For this review, use the dimensioned drawing (mm, ordinates from the lowest corner) and the shaded views. A direction names the side the tool comes from. Round coordinates to 2 decimals unless told otherwise and drop trailing zeros. Write each loop counter-clockwise with the first axis right and the second up, starting at its lowest first coordinate (ties: lowest second). Pieces come first, ordered by that corner, then holes. Notation, with made-up numbers: M 5,-21 L 57,-21 A17 cw 57,5 Z; hole C 70,34 d4. An arc over 180 degrees is marked long. Write each question's results on one line, items separated by ' | '. Start each with the question number.
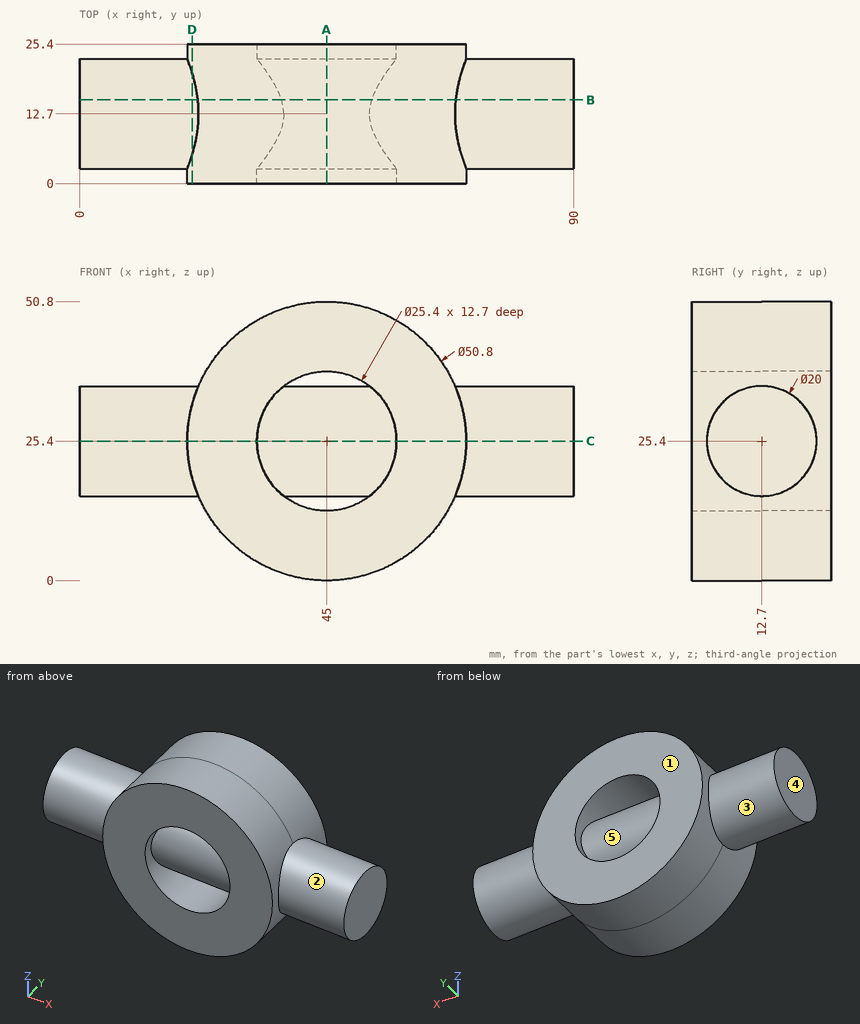
Item 1: We need section A-A on x = 45. State the section outline as (y, z) points, then the cut area to 3 significant figures.
Item 2: We need section C-C on z = 25.4. State the section outline as (x, y) points.
Item 3: For probe 1 along Z at (x, y) = (45, 22.75); probe 2 along Z at (x, y) = (45, 4); probe 3 along Z at (x, y) = (23, 17.75), list the stretches that pass through material, from the lowest coordinate up.
Item 4: We need section B-B on y = 15.25. State the section outline as (x, z) points, then the cut area to 3 significant figures.
Item 5: For the marked faces 1 and 2, list the 3-axis set-ups (+Z, -Z, +X, -X, +Y, -Y) from which the entire face can be reached by the end or side of a thin tool; tool diameter is ignored.
Item 6: Mouldability with a two-part tool opening along Z and no side actions: class the marked faces 3, 4 and 5 as pulls with the +Z half, pulls with the -Z half, needs draft (parallel to the pull), parting line crosses it, or undercut.
Item 7: We need section D-D on x = 20.5. State the section outline as (y, z) points, then the cut area to 3 significant figures.
Item 8: Insertion check: P1, Ø6, axis at y = 9.5, z = 8.5, coming from the +X side; P2, Ø23, axis at x = 45, z = 25.4, coming from the -Y side; P3, Ø6, axis at y = 10, z = 11, coming from the -X side. Each pin has a flat end and moves straight along its axis. Give the tip position at first contact, or say it passes through.
Numbers:
1) outline: M 0,0 L 25.4,0 L 25.4,12.7 L 0,12.7 Z; M 0,38.1 L 25.4,38.1 L 25.4,50.8 L 0,50.8 Z; C 12.7,25.4 d20 | area: 959 mm^2
2) outline: M 0,2.7 L 19.6,2.7 L 19.6,0 L 32.3,0 L 32.3,2.7 L 57.7,2.7 L 57.7,0 L 70.4,0 L 70.4,2.7 L 90,2.7 L 90,22.7 L 70.4,22.7 L 70.4,25.4 L 57.7,25.4 L 57.7,22.7 L 32.3,22.7 L 32.3,25.4 L 19.6,25.4 L 19.6,22.7 L 0,22.7 Z
3) probe 1: z = 0 to 12.7, 38.1 to 50.8 | probe 2: z = 0 to 12.7, 20.47 to 30.33, 38.1 to 50.8 | probe 3: z = 12.71 to 38.09
4) outline: M 0,15.73 L 21.51,15.73 A25.4 ccw 68.49,15.73 L 90,15.73 L 90,35.07 L 68.49,35.07 A25.4 ccw 21.51,35.07 L 0,35.07 Z; hole M 36.77,15.73 A12.7 ccw 53.23,15.73 Z; hole M 36.77,35.07 L 53.23,35.07 A12.7 ccw Z | area: 2,740 mm^2
5) face 1: +Z, -Z, +X, -X, +Y | face 2: +X
6) face 3: parting line crosses it | face 4: needs draft | face 5: undercut
7) outline: M 0,18.7 L 5.28,18.7 A10 ccw 20.12,18.7 L 25.4,18.7 L 25.4,32.1 L 20.12,32.1 A10 ccw 5.28,32.1 L 0,32.1 Z | area: 408 mm^2
8) P1: stops at x = 66.26 | P2: stops at y = 2.7 | P3: stops at x = 22.3
